```python
from build123d import *

# Parameters (mm, degrees)
SKETCH_3_W      = 0.91875
SKETCH_3_H      = 15
SKETCH_3_R      = 1.8
EXTRUDE_2_DEPTH = 2


with BuildPart() as part:
    # 草图3 → 凸台-拉伸2 (new body)
    with BuildSketch(Plane(origin=(0, 0, 0), x_dir=(1, 0, 0), z_dir=(0, 1, 0))):
        Polygon((8.65, -21.5), (20.65, -21.5), (20.65, -27), (27, -27), (27, 27), (-27, 27), (-27, -27), (8.65, -27), align=None)
        with Locations((-10.896875, -5.8)):
            Rectangle(SKETCH_3_W, SKETCH_3_H, mode=Mode.SUBTRACT)
        with Locations((-8.140625, -5.8)):
            Rectangle(SKETCH_3_W, SKETCH_3_H, mode=Mode.SUBTRACT)
        with Locations((-5.384375, -5.8)):
            Rectangle(SKETCH_3_W, SKETCH_3_H, mode=Mode.SUBTRACT)
        with Locations((-2.628125, -5.8)):
            Rectangle(SKETCH_3_W, SKETCH_3_H, mode=Mode.SUBTRACT)
        with Locations((0.128125, -5.8)):
            Rectangle(SKETCH_3_W, SKETCH_3_H, mode=Mode.SUBTRACT)
        with Locations((2.884375, -5.8)):
            Rectangle(SKETCH_3_W, SKETCH_3_H, mode=Mode.SUBTRACT)
        with Locations((5.640625, -5.8)):
            Rectangle(SKETCH_3_W, SKETCH_3_H, mode=Mode.SUBTRACT)
        with Locations((8.396875, -5.8)):
            Rectangle(SKETCH_3_W, SKETCH_3_H, mode=Mode.SUBTRACT)
        with Locations((23.5, 23.5)):
            Circle(SKETCH_3_R, mode=Mode.SUBTRACT)
        with Locations((23.5, -23.5)):
            Circle(SKETCH_3_R, mode=Mode.SUBTRACT)
        with Locations((-23.5, 23.5)):
            Circle(SKETCH_3_R, mode=Mode.SUBTRACT)
        with Locations((-23.5, -23.5)):
            Circle(SKETCH_3_R, mode=Mode.SUBTRACT)
    extrude(amount=EXTRUDE_2_DEPTH)


solid = part.part
```
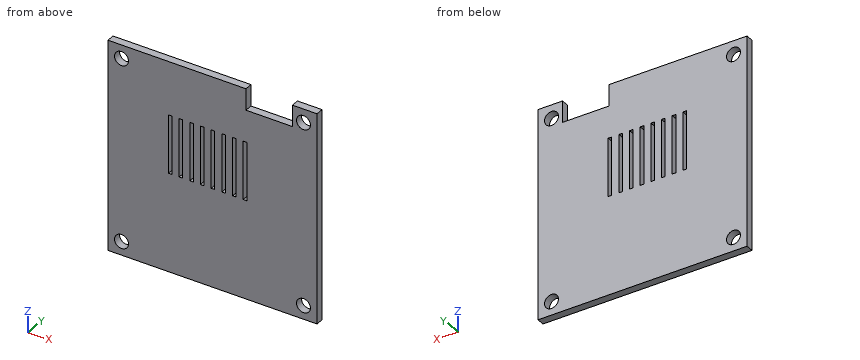
Source: CAD feature listing. Evaluate the final solid. Frame: model axes, mm. Round coordinates to 2 decimals unless told otherwise and drop trailing zeros. Order: outer loops, then holes, each group sorted by start corner. A loop starts at its lowest first (then second) coordinate and runs counter-clockwise, first axis right, second up. Notation, with made-up numbers: (22, -4.75) -> (56, -4.75) arc R18 ccw to (56, 7.25) -> close; hole circle Ø3 at (-23, 0). An arc over 180 degrees is marked (long way). One line per item, written item: value. Start each with the question number.
Q1. Pin query (flat end, axial travel): pin 1 (2 mm diameter, centred on x = -15.5, z = 2.5, fed in from -Y). Return the tip coordinate at first contact, or that it passes through.
Q2. Section query A-A (x = 23.5). Return the cut outline in (y, z).
Q3. Section query C-C (z = 23.5). Return the cut outline in (x, y), plus the area to 3 significant figures.
Q4. Material intervals for probe 1 along X at (y, z) = (1.25, -23.5); probe 2 along X at (y, z) = (1, 23.5), sorted ascending.
Q5. Section query B-B (z = -23.5). Return the cut outline in (x, y), plus the area to 3 significant figures.
Q6. Section query D-D (y = 0.75). Give the number of separate pieces and of enclosed holes in the cut face, plus the area to 3 significant figures.
Findings below:
1. pin 1: y = 0
2. outline: (0, -27) -> (2, -27) -> (2, -25.3) -> (0, -25.3) -> close; (0, -21.7) -> (2, -21.7) -> (2, 21.7) -> (0, 21.7) -> close; (0, 25.3) -> (2, 25.3) -> (2, 27) -> (0, 27) -> close
3. outline: (-27, 0) -> (-25.3, 0) -> (-25.3, 2) -> (-27, 2) -> close; (-21.7, 0) -> (8.65, 0) -> (8.65, 2) -> (-21.7, 2) -> close; (20.65, 0) -> (21.7, 0) -> (21.7, 2) -> (20.65, 2) -> close; (25.3, 0) -> (27, 0) -> (27, 2) -> (25.3, 2) -> close
3. area: 69.6 mm²
4. probe 1: -27 to -25.3, -21.7 to 21.7, 25.3 to 27
4. probe 2: -27 to -25.3, -21.7 to 8.65, 20.65 to 21.7, 25.3 to 27
5. outline: (-27, 0) -> (-25.3, 0) -> (-25.3, 2) -> (-27, 2) -> close; (-21.7, 0) -> (21.7, 0) -> (21.7, 2) -> (-21.7, 2) -> close; (25.3, 0) -> (27, 0) -> (27, 2) -> (25.3, 2) -> close
5. area: 93.6 mm²
6. separate pieces: 1
6. enclosed holes: 12
6. area: 2,700 mm²
